Could you check a few things on this model? Use its own coordinates, in mm. Round coordinates to 2 decimals unless told otherwise and drop trailing zeros. Write each loop counter-clockwise with the first axis right and the second up, starting at its lowest first coordinate (ties: lowest second). Pieces come first, ordered by that corner, then holes.
Autodesk Inventor part; units mm, degrees
ref_plane "YZ Plane" through (0, 0, 0) normal (1, 0, 0) x (0, 1, 0)
ref_plane "XZ Plane" through (0, 0, 0) normal (0, 1, 0) x (-1, 0, 0)
ref_plane "XY Plane" through (0, 0, 0) normal (0, 0, 1) x (1, 0, 0)
sketch "Sketch1" plane through (0, 0, 0) normal (0, 0, 1) x (1, 0, 0)
  line L0 (-12, 106.1721) -> (1464, 106.1721)
  line L1 (1464, 106.1721) -> (1464, 406.1721)
  line L2 (1464, 406.1721) -> (-12, 406.1721)
  line L3 (-12, 406.1721) -> (-12, 106.1721)
  line L4 (-12, 406.1721) -> (18, 406.1721)
  line L5 (1464, 406.1721) -> (1446, 406.1721)
  line L6 (1446, 256.1721) -> (1464, 256.1721)
  line L7 (1464, 256.1721) -> (1464, 406.1721)
  line L8 (1446, 256.1721) -> (1446, 106.1721)
  line L9 (-12, 106.1721) -> (6, 106.1721)
  line L10 (6, 106.1721) -> (6, 256.1721)
  line L11 (6, 256.1721) -> (-12, 256.1721)
  line L12 (-12, 256.1721) -> (-12, 106.1721)
  point P0 (0, 0)
  point P1 (18, 106.1721)
  dimension "d1" = 1476
  dimension "d2" = 300
  dimension "d5" = 18
  dimension "d6" = 150
  dimension "d35" = 18
  dimension "d36" = 150
extrude "Extrusion1" add sketch "Sketch1" along normal blind 18 contours L3 L11 L10 L0 | L10 L11 L3 L2 L1 L6 L8 L0
sketch "Sketch2" plane through (-12, 256.1721, 0) normal (-1, 0, 0) x (0, 0, 1)
  line L0 (0, 0) -> (0, 150)
  line L1 (0, 150) -> (9, 150)
  line L2 (18, 0) -> (18, 150)
  line L3 (0, 150) -> (9, 150) construction
  line L4 (0, 150) -> (18, 150)
  line L5 (9, 150) -> (168.25, 150) construction
  line L6 (9, 150) -> (168.25, 150) construction
  line L7 (0, -150) -> (0, 0)
  line L8 (9, -9.25) -> (59, -9.25) construction
  circle A0 centre (9, -59.25) radius 2.5
  circle A1 centre (9, 40.75) radius 2.5
  circle A2 centre (9, -9.25) radius 2.5
  point P0 (0, -256.1721)
  dimension "d10" = 0
  dimension "d16" = 159.25
  dimension "d21" = 5
  dimension "d22" = 5
  dimension "d23" = 5
sketch "Sketch3" plane through (1464, 256.1721, 0) normal (1, 0, 0) x (0, 0, -1)
  line L0 (0, 0) -> (0, 150)
  line L1 (0, 150) -> (-9, 150)
  circle A0 centre (-9, 40.75) radius 2.5
  circle A1 centre (-9, -9.25) radius 2.5
  circle A2 centre (-9, -59.25) radius 2.5
  point P0 (0, -256.1721)
  dimension "d24" = 9
  dimension "d28" = 5
  dimension "d29" = 5
  dimension "d30" = 5
extrude "Extrusion2" cut sketch "Sketch3" against normal blind 42
extrude "Extrusion3" cut sketch "Sketch2" against normal blind 42
sketch "Sketch4" plane through (0, 0, 0) normal (0, 0, -1) x (-1, 0, 0)
  line L0 (12, 106.1721) -> (-1446, 106.1721)
  line L1 (12, 106.1721) -> (-6, 106.1721)
  line L2 (-6, 106.1721) -> (-6, 256.1721)
  line L3 (-6, 256.1721) -> (12, 256.1721)
  line L4 (12, 256.1721) -> (12, 106.1721)
  point P0 (0, 0)
  dimension "d39" = 18
  dimension "d40" = 150
extrude "Extrusion4" cut sketch "Sketch4" against normal blind 208.825
sketch "Sketch5" plane through (0, 0, 0) normal (0, 0, -1) x (-1, 0, 0)
  line L0 (-1446, 256.1721) -> (-1464, 256.1721)
  line L1 (-6, 256.1721) -> (379, 256.1721) construction
  circle A0 centre (-396, 331.1721) radius 50
  point P0 (0, 0)
  dimension "d53" = 100
extrude "Extrusion5" cut sketch "Sketch5" against normal blind 208.825
properties part number "reardraws" material "MDF Medium Density Fiberboard"
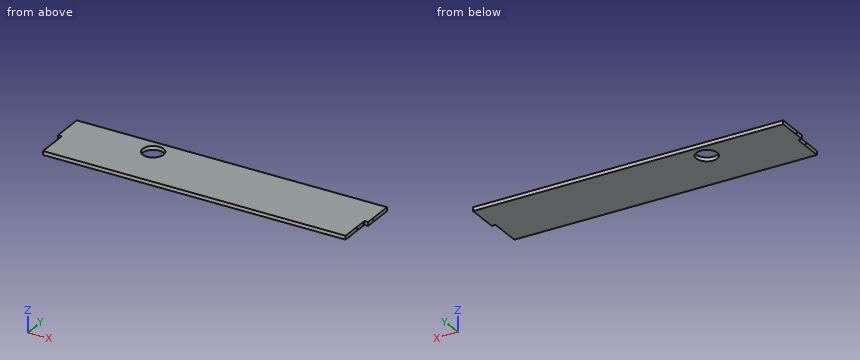
Q1. Imagine slicing it at C-C, the plane z = 3.25. Write out the boundary of the cut face in (x, y).
Q2. Imagine slicing it at D-D, the plane y = 216.5. Write out the boundary of the cut face in (x, z), then the cut area to 3 significant figures.
Q3. If I drill on L1, parallel to Y at x = 13.25, z = 9; L2, parallel to Y at x = 396, z = 5.75; L3, parallel to X at y = 329, z = 6, over which ranges is the centre line in solid material (lowest first)?
Q4. Imagine slicing it at A-A, the plane x = 396. Write out the boundary of the cut face in (y, z), then the cut area to 3 significant figures.
Q5. I'm going to push flat-ended pins straight in: pin 1 Ø1.5 at (y, z) = (196, 8) entering from -X; pin 2 Ø1.5 at (y, z) = (296.5, 9) entering from +X; pin 3 Ø3 at (y, z) = (153.5, 9.5) entering from +X. Where does each tip first touch, or does it pass through?
Q6. Imagine slicing it at B-B, the plane y = 357. Write out the boundary of the cut face in (x, z), then the cut area to 3 significant figures.
Results found:
1. outline: (-12, 256.17) - (6, 256.17) - (6, 106.17) - (1446, 106.17) - (1446, 256.17) - (1464, 256.17) - (1464, 406.17) - (-12, 406.17) - close; hole circle Ø100 at (396, 331.17)
2. outline: (6, 0) - (1446, 0) - (1446, 18) - (6, 18) - close
2. area: 25,900 mm2
3. L1: y = 106.17 to 194.42, 199.42 to 244.42, 249.42 to 294.42, 299.42 to 406.17
3. L2: y = 106.17 to 281.17, 381.17 to 406.17
3. L3: x = -12 to 346.05, 445.95 to 1464
4. outline: (106.17, 0) - (281.17, 0) - (281.17, 18) - (106.17, 18) - close; (381.17, 0) - (406.17, 0) - (406.17, 18) - (381.17, 18) - close
4. area: 3,600 mm2
5. pin 1: stops at x = 30
5. pin 2: stops at x = 1422
5. pin 3: stops at x = 1446
6. outline: (-12, 0) - (353.19, 0) - (353.19, 18) - (-12, 18) - close; (438.81, 0) - (1464, 0) - (1464, 18) - (438.81, 18) - close
6. area: 25,000 mm2
